Geometry: see drawing. Coordinates: mm, zero at the bounding-box minimum. Give positions to 0.01 mm unless a question says otherwise; leave off trailing zeros. Order: outer loops, then holes, each group sorted by start corner. A loop starts at its lowest first (then second) coordinate and runs counter-clockwise, first axis right, second up. Notation, with made-up numbers: M 71.5,-36.75 L 92.5,-36.75 A20 cw 92.5,-16.75 Z; hole C 38.5,20 d2. An arc over 180 degrees is marked long. Write item = value, one per line. Start each with the question number.
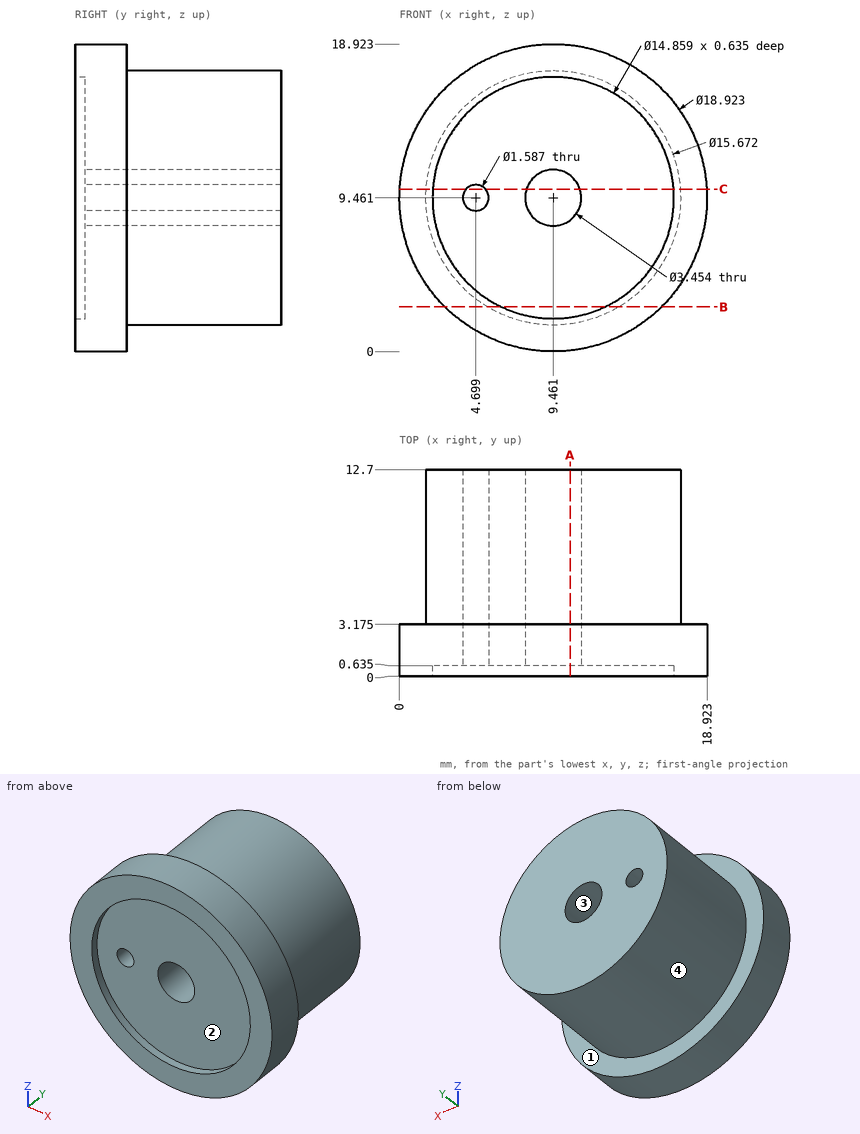
1) Cut plane C-C (z = 10). Return loops of the section in (x, y) (1 decimal), plus the area to 3 significant figures.
2) Cut plane B-B (z = 2.75). Return loops of the section in (x, y) (1 decimal), plus the area to 3 significant figures.
3) Cut plane A-A (x = 10.5). Return loops of the section in (y, z) (1 decimal), plus the area to 3 significant figures.
4) Ray query, L1, parallel to Y at x = 17.25, z = 12.25 (1 decimal); L2, parallel to Y at x = 11.5, z = 14.5 (1 decimal); L3, parallel to Z at x = 8.5, y = 9.75 (1 decimal). Return the intervals inside material, ascending.
5) Pin query (flat end, axial travel): pin 1 Ø2 at (x, z) = (4.7, 9.46) entering from +Y; pin 2 Ø3 at (x, y) = (3.5, 10) entering from -Z; pin 3 Ø5 at (y, z) = (8.5, 8.5) entering from +X; pin 4 Ø4 at (x, y) = (6.5, 11.5) entering from -Z (1 decimal). Return the tip coordinate at first contact, or that it passes through.
6) Draft query along X for the marked faces 1, 2, 3 and 4. Return one class per face: pulls with the +X half, pulls with the -X half, needs draft (parallel to the pull), parting line crosses it, or undercut.
Reply:
q1.outline = M 0,0 L 2.1,0 L 2.1,0.6 L 4.1,0.6 L 4.1,12.7 L 1.6,12.7 L 1.6,3.2 L 0,3.2 Z; M 5.3,0.6 L 7.8,0.6 L 7.8,12.7 L 5.3,12.7 Z; M 11.1,0.6 L 16.9,0.6 L 16.9,0 L 18.9,0 L 18.9,3.2 L 17.3,3.2 L 17.3,12.7 L 11.1,12.7 Z
q1.area = 146 mm²
q2.outline = M 2.8,0 L 6.3,0 L 6.3,0.6 L 12.6,0.6 L 12.6,0 L 16.1,0 L 16.1,3.2 L 13.5,3.2 L 13.5,12.7 L 5.4,12.7 L 5.4,3.2 L 2.8,3.2 Z
q2.area = 115 mm²
q3.outline = M 0,0.1 L 3.2,0.1 L 3.2,1.7 L 12.7,1.7 L 12.7,8.1 L 0.6,8.1 L 0.6,2.1 L 0,2.1 Z; M 0,16.8 L 0.6,16.8 L 0.6,10.8 L 12.7,10.8 L 12.7,17.2 L 3.2,17.2 L 3.2,18.9 L 0,18.9 Z
q3.area = 165 mm²
q4.L1 = 0 to 3.2
q4.L2 = 0.6 to 12.7
q4.L3 = 1.7 to 8, 10.9 to 17.2
q5.pin_1 = 12.7
q5.pin_2 = 3.02
q5.pin_3 = 17.3
q5.pin_4 = 1.7
q6.face_1 = needs draft
q6.face_2 = undercut
q6.face_3 = undercut
q6.face_4 = parting line crosses it
